For this review, take the finished solid that the model builds, in its own axes (mm). A direction names the side the tool comes from. Round coordinates to 2 decimals unless told otherwise and drop trailing zeros. Order: outer loops, then holes, each group sorted by start corner. A loop starts at its lowest first (then second) coordinate and runs counter-clockwise, first axis right, second up. Notation, with made-up numbers: (0, 63.5) - (22, 63.5) arc R22 cw to (22, 81.5) - close; hole circle Ø5 at (-17, 3). An arc over 180 degrees is marked (long way). One line per question, with ' | ' between items.
```python
from build123d import *

# Parameters (mm, degrees)
SALIENTE_EXTRUIR1_DEPTH   = 5
SALIENTE_EXTRUIR1_2_DEPTH = 5
SALIENTE_EXTRUIR1_3_DEPTH = 5
SALIENTE_EXTRUIR1_4_DEPTH = 5
CROQUIS3_W                = 20
CROQUIS3_H                = 20
SALIENTE_EXTRUIR2_DEPTH   = 5
REDONDEO1_R               = 2


with BuildPart() as part:
    # Croquis2 → Saliente-Extruir1 (new body)
    with BuildSketch(Plane(origin=(0, 0, 0), x_dir=(1, 0, 0), z_dir=(0, 1, 0))):
        Polygon((-3.880962474, 9.7), (-4.31520152, 10), (4.31520152, 10), (3.880962474, 9.7), (3.100109842, 9.007732001), (3.100109842, 7.886854264), (5.174607071, 7.886854264), (5.174607071, 6.657084853), (2.689193029, 4.171670811), (-2.689193029, 4.171670811), (-5.174607071, 6.657084853), (-5.174607071, 7.886854264), (-3.100109842, 7.886854264), (-3.100109842, 9.007732001), align=None)
    extrude(amount=SALIENTE_EXTRUIR1_DEPTH)



with BuildPart() as body_2:
    # Croquis2 → Saliente-Extruir1 2 (new body)
    with BuildSketch(Plane(origin=(0, 0, 0), x_dir=(1, 0, 0), z_dir=(0, 1, 0))):
        Polygon((10, 4.31520152), (10, -4.31520152), (9.7, -3.880962474), (9.007732001, -3.100109842), (7.886854264, -3.100109842), (7.886854264, -5.174607071), (6.657084853, -5.174607071), (4.171670811, -2.689193029), (4.171670811, 2.689193029), (6.657084853, 5.174607071), (7.886854264, 5.174607071), (7.886854264, 3.100109842), (9.007732001, 3.100109842), (9.7, 3.880962474), align=None)
    extrude(amount=SALIENTE_EXTRUIR1_2_DEPTH)


with BuildPart() as body_3:
    # Croquis2 → Saliente-Extruir1 3 (new body)
    with BuildSketch(Plane(origin=(0, 0, 0), x_dir=(1, 0, 0), z_dir=(0, 1, 0))):
        Polygon((4.31520152, -10), (-4.31520152, -10), (-3.880962474, -9.7), (-3.100109842, -9.007732001), (-3.100109842, -7.886854264), (-5.174607071, -7.886854264), (-5.174607071, -6.657084853), (-2.689193029, -4.171670811), (2.689193029, -4.171670811), (5.174607071, -6.657084853), (5.174607071, -7.886854264), (3.100109842, -7.886854264), (3.100109842, -9.007732001), (3.880962474, -9.7), align=None)
    extrude(amount=SALIENTE_EXTRUIR1_3_DEPTH)


with BuildPart() as body_4:
    # Croquis2 → Saliente-Extruir1 4 (new body)
    with BuildSketch(Plane(origin=(0, 0, 0), x_dir=(1, 0, 0), z_dir=(0, 1, 0))):
        Polygon((-10, -4.31520152), (-10, 4.31520152), (-9.7, 3.880962474), (-9.007732001, 3.100109842), (-7.886854264, 3.100109842), (-7.886854264, 5.174607071), (-6.657084853, 5.174607071), (-4.171670811, 2.689193029), (-4.171670811, -2.689193029), (-6.657084853, -5.174607071), (-7.886854264, -5.174607071), (-7.886854264, -3.100109842), (-9.007732001, -3.100109842), (-9.7, -3.880962474), align=None)
    extrude(amount=SALIENTE_EXTRUIR1_4_DEPTH)


with BuildPart() as part_1:
    add(part.part)

    add(body_2.part)  # Saliente-Extruir2 merges body 2

    add(body_3.part)  # Saliente-Extruir2 merges body 3

    add(body_4.part)  # Saliente-Extruir2 merges body 4
    # Croquis3 → Saliente-Extruir2 (add)
    with BuildSketch(Plane(origin=(0, 5, 0), x_dir=(1, 0, 0), z_dir=(0, 1, 0))):
        Rectangle(CROQUIS3_W, CROQUIS3_H)
    extrude(amount=SALIENTE_EXTRUIR2_DEPTH)

    # Redondeo1
    redondeo1_edges = [part_1.edges().sort_by_distance(p)[0] for p in [
        (10, 10, 0),
        (0, 10, -10),
        (-10, 10, 0),
        (0, 10, 10),
    ]]
    fillet(redondeo1_edges, radius=REDONDEO1_R)


solid = part_1.part
```
(1) Mouldability with a two-part tool opening along Z and no side actions: class faces 4 (the flat face through (0, 0, -7)), 5 (the cylindrical face through (0.14, 9.4, -9.43)), 6 (the flat face through (-4, 2, -7.887)) as released by +Z, released by -Z, zero draft, split by the parting line, or undercut.
Output values:
face 4: zero draft | face 5: released by -Z | face 6: undercut
(2) For faces 1 (the flat face through (4, 2, 7.887)), 2 (the flat face through (-5.175, 2, -7)), 3 (the flat face through (5.175, 2, -7)), list the 3-axis set-ups (+Z, -Z, +X, -X, +Y, -Y) from which the entire face can be reached by the end or side of a thin tool; tool diameter is ignored.
Output values:
face 1: +X, -Y | face 2: -Z, -X, -Y | face 3: -Z, +X, -Y
(3) We need section D-D on y = 9.25. State the section outline as (x, z) points.
Output values:
outline: (-9.56, -9.56) - (9.56, -9.56) - (9.56, 9.56) - (-9.56, 9.56) - close
(4) We need section A-A on x = -7. State the section outline as (y, z) points.
Output values:
outline: (0, -5.17) - (5, -5.17) - (5, -10) - (8, -10) arc R2 ccw to (10, -8) - (10, 8) arc R2 ccw to (8, 10) - (5, 10) - (5, 5.17) - (0, 5.17) - close
(5) Insertion check: pin 1 (0.6 mm diameter, centred on x = -8.5, y = 3, fed in from +Z); pin 2 (1.5 mm diameter, centred on x = 1, z = 0, fed in from -Y); pin 3 (0.6 mm diameter, centred on y = 3.5, z = -7.5, fed in from +X). Each pin has a flat end and moves straight along its axis. Give the tip position at first contact, or say it passes through.
Output values:
pin 1: z = 3.1 | pin 2: y = 5 | pin 3: x = 5.17
(6) We need section B-B on z = 7.5. State the section outline as (x, y) points, plus the area to 3 significant figures.
Output values:
outline: (-10, 5) - (-5.17, 5) - (-5.17, 0) - (5.17, 0) - (5.17, 5) - (10, 5) - (10, 8) arc R2 ccw to (8, 10) - (-8, 10) arc R2 ccw to (-10, 8) - close | area: 150 mm^2
(7) We need section C-C on y = 2.75. Give the number of separate pieces and of enclosed holes in the cut face, plus the area to 3 significant figures.
Output values:
separate pieces: 4 | enclosed holes: 0 | area: 186 mm^2
(8) For probe 1 along X at (y, z) = (3, -2.5); probe 2 along Z at (x, y) = (-4, 0.5), list the stretches that pass through material, from the lowest coordinate up. Write a range as [from, to].
Output values:
probe 1: [-10, -4.17], [4.17, 10] | probe 2: [-10, -9.78], [-7.89, -5.48], [5.48, 7.89], [9.78, 10]
